Read the model definition and answer for the solid it produces. Units are mm, in the model's axes. A direction names the side the tool comes from. Coordinates: 2 decimals unless noted, no trailing zeros. Write each loop counter-clockwise with the first axis right and the second up, starting at its lowest first coordinate (ties: lowest second). Pieces come first, ordered by that corner, then holes. Notation, with made-up numbers: (21, -39) -> (38, -39) arc R17 ccw to (38, -12) -> close; hole circle Ø10 at (14.5, -0.75). An arc over 180 degrees is marked (long way). Return JSON: item names as keys, results as strings.
from build123d import *


with BuildPart() as part:
    # Schizzo1 → Rivoluzione1 (revolve)
    with BuildSketch(Plane.XY, mode=Mode.PRIVATE) as rivoluzione1_sk:
        with BuildLine():
            Line((0, 66.166666667), (0, 55))
            Line((0, 55), (4, 55))
            Line((4, 55), (7.2, 52.5))
            Line((7.2, 52.5), (10.8, 56.25))
            Line((10.8, 56.25), (10.8, 57.5))
            Line((10.8, 57.5), (9.6, 57.5))
            ThreePointArc((9.6, 57.5), (7.2, 59.9), (4.8, 57.5))
            Line((4.8, 57.5), (4, 57.5))
            Line((4, 57.5), (4, 62.5))
            Line((4, 62.5), (12, 62.5))
            Line((12, 62.5), (12, 66.833333333))
            ThreePointArc((12, 66.833333333), (11.804737854, 67.304737854), (11.333333333, 67.5))
            Line((11.333333333, 67.5), (1.333333333, 67.5))
            ThreePointArc((1.333333333, 67.5), (0.390524292, 67.109475708), (0, 66.166666667))
        make_face()
    revolve(rivoluzione1_sk.sketch.rotate(Axis((11.333333333, 0, 0), (-1, 0, 0)), 270), axis=Axis((11.333333333, 0, 0), (-1, 0, 0)))


solid = part.part
1. For a pull along Z with two mould halves and no side action, classify faces 1 (the face through (2.028, -48.794, 25.379)), 2 (the face through (0, 49.3, -24.8)), 3 (the face through (10.192, -56.133, -12.465)), 4 (the face through (6.263, -59.884, 31.147)) as +Z half, -Z half, draft (parallel to the pull), parting line (faces both ways), or undercut.
Taken from the geometry:
{"face 1": "undercut", "face 2": "draft", "face 3": "undercut", "face 4": "parting line"}
2. Consider L1, parallel to Y at x = 1.45, z = 0; L2, parallel to Y at x = 8.75, z = 32.5; L3, parallel to Z at x = 5.25, y = -7. Determine where each line is inside the solid, lowest interval first.
Taken from the geometry:
{"L1": "y = -67.5 to -55, 55 to 67.5", "L2": "y = -59.16 to -53.39, -49.64 to -43.27, 43.27 to 49.64, 53.39 to 59.16", "L3": "z = -67.14 to -62.11, -58.48 to -53.57, 53.57 to 58.48, 62.11 to 67.14"}
3. Flat-ended cylindrical pins translate along their axes: pin 1 Ø1.5 at (x, z) = (6.5, 16) entering from +Y; pin 2 Ø3 at (x, z) = (6, -46.5) entering from +Y; pin 3 Ø5 at (x, y) = (1, 16.5) entering from +Z. Find the tip coordinate at first contact, or state that the pin passes through.
Taken from the geometry:
{"pin 1": "stops at y = 65.75", "pin 2": "stops at y = 50.31", "pin 3": "stops at z = 66.03"}
4. The part is cut by section A-A (y = 0). Determine the outline of the cut face in (x, z), then the cut area to 3 significant figures.
Taken from the geometry:
{"outline": "(0, -66.17) arc R1.33 ccw to (1.33, -67.5) -> (11.33, -67.5) arc R0.67 ccw to (12, -66.83) -> (12, -62.5) -> (4, -62.5) -> (4, -57.5) -> (4.8, -57.5) arc R2.4 ccw to (9.6, -57.5) -> (10.8, -57.5) -> (10.8, -56.25) -> (7.2, -52.5) -> (4, -55) -> (0, -55) -> close; (0, 55) -> (4, 55) -> (7.2, 52.5) -> (10.8, 56.25) -> (10.8, 57.5) -> (9.6, 57.5) arc R2.4 ccw to (4.8, 57.5) -> (4, 57.5) -> (4, 62.5) -> (12, 62.5) -> (12, 66.83) arc R0.67 ccw to (11.33, 67.5) -> (1.33, 67.5) arc R1.33 ccw to (0, 66.17) -> close", "area": "244 mm2"}
5. A tool of negligible diameter and unlimited length cuts with its end or side. For faces 5 (the face through (7.045, 15.806, 50.191)), 6 (the face through (4, -51, -27)), 7 (the face through (10.8, -38, -42)), from which of +Z, -Z, +X, -X, +Y, -Y can it reach the whole face along a straight path? Write none if from no direction.
Taken from the geometry:
{"face 5": "-X", "face 6": "none", "face 7": "+X"}
